```python
from build123d import *

# Parameters (mm, degrees)
BOSS_EXTRUDE1_DEPTH = 152.4
BOSS_EXTRUDE2_DEPTH = 173.99
CUT_EXTRUDE1_DEPTH  = 232.798485112
BOSS_EXTRUDE3_DEPTH = 2.54
CUT_EXTRUDE2_DEPTH  = 247.386546305
FILLET1_R           = 2.54


with BuildPart() as part:
    # Sketch1 → Boss-Extrude1 (new body)
    with BuildSketch(Plane.XY):
        Polygon((0, 0), (-173.99, 0), (-158.75, 15.24), (-152.4, 15.24), (-152.4, 2.54), (0, 2.54), align=None)
    extrude(amount=BOSS_EXTRUDE1_DEPTH)

    # Sketch2 → Boss-Extrude2 (add, through all)
    with BuildSketch(Plane(origin=(0, 0, 0), x_dir=(0, 0, -1), z_dir=(1, 0, 0))):
        Polygon((-152.4, 2.54), (-152.4, 15.24), (-158.75, 15.24), (-173.99, 0), (-152.4, 0), align=None)
    extrude(amount=-BOSS_EXTRUDE2_DEPTH)

    # Sketch3 → Cut-Extrude1 (cut, through all)
    with BuildSketch(Plane(origin=(0, 0, 152.4), x_dir=(-1, 0, 0), z_dir=(0, 0, -1))):
        Polygon((158.75, 15.24), (173.99, 0), (173.99, 15.24), align=None)
    extrude(amount=-CUT_EXTRUDE1_DEPTH, mode=Mode.SUBTRACT)

    # Sketch4 → Boss-Extrude3 (add, through all)
    with BuildSketch(Plane(origin=(0, 2.54, 0), x_dir=(1, 0, 0), z_dir=(0, 1, 0))):
        with BuildLine():
            ThreePointArc((-105.230385896, 0), (-114.3, 21.59), (-123.369614104, 0))
            Line((-123.369614104, 0), (-105.230385896, 0))
        make_face()
        with BuildLine():
            ThreePointArc((0, -47.169614104), (21.59, -38.1), (0, -29.030385896))
            Line((0, -29.030385896), (0, -47.169614104))
        make_face()
    extrude(amount=-BOSS_EXTRUDE3_DEPTH)

    # Sketch4<3> → Cut-Extrude2 (cut, through all)
    with BuildSketch(Plane(origin=(0, 2.54, 0), x_dir=(1, 0, 0), z_dir=(0, 1, 0))):
        with BuildLine():
            Line((-29.030385896, 0), (-47.169614104, 0))
            ThreePointArc((-47.169614104, 0), (-38.1, -21.59), (-29.030385896, 0))
        make_face()
        with BuildLine():
            Line((0, -123.369614104), (0, -105.230385896))
            ThreePointArc((0, -105.230385896), (-21.59, -114.3), (0, -123.369614104))
        make_face()
    extrude(amount=-CUT_EXTRUDE2_DEPTH, mode=Mode.SUBTRACT)

    # Fillet1
    fillet1_edges = [part.edges().sort_by_distance(p)[0] for p in [
        (-123.369614104, 1.27, 0),
        (-105.230385896, 1.27, 0),
        (0, 1.27, 29.030385896),
        (0, 1.27, 47.169614104),
        (-47.169614104, 1.27, 0),
        (-29.030385896, 1.27, 0),
        (0, 1.27, 105.230385896),
        (0, 1.27, 123.369614104),
    ]]
    fillet(fillet1_edges, radius=FILLET1_R)


solid = part.part
```
Geometry: final body of the model. Coordinates: model frame, mm. A direction names the side the tool comes from. Coordinates: 2 decimals unless noted, no trailing zeros. Order: outer loops, then holes, each group sorted by start corner. A loop starts at its lowest first (then second) coordinate and runs counter-clockwise, first axis right, second up.
Item 1: Access query for faces 1 (the face through (0, 6, 156)), 2 (the face through (-156, 6, 0)), 3 (the face through (21.585, 1.288, 38.456)), 4 (the face through (-152.4, 9, 75)). Directions: +Z, -Z, +X, -X, +Y, -Y. A direction counts if a zero-diameter tool reaches every point of the face in a straight line with its end or side. Return the directions, or none.
Answer:
face 1: +Z, +X, +Y, -Y
face 2: -Z, -X, +Y, -Y
face 3: +Y, -Y
face 4: -Z, +X, +Y
Item 2: Contact query for flat-ended pins moving along their axis: P1, Ø6, axis at x = -33.5, y = 8.5, coming from the +Z side; P2, Ø7.5, axis at x = -161, y = 11.5, coming from the -Z side; P3, Ø0.8, axis at y = 1, z = 77.5, coming from the +X side. Output: stop coordinate, or through.
Answer:
P1: stops at z = 168.49
P2: stops at z = 0
P3: stops at x = 0
Item 3: Section query D-D (z = 38.1). Output: boundary loops of the cut face in (x, y), then the cut area to 3 significant figures.
Answer:
outline: (-173.99, 0) - (21.59, 0) - (21.59, 2.54) - (-152.4, 2.54) - (-152.4, 15.24) - (-158.75, 15.24) - close
area: 655 mm2
Item 4: Material intervals for line 1 along Y through (x, z) = (-1, 39); line 2 along X through (y, z) = (1.35, 8.89); line 3 along Z through (x, y) = (-126, 2.5), sorted ascending.
Answer:
line 1: y = 0 to 2.54
line 2: x = -172.64 to -50.8, -25.4 to 0
line 3: z = -13.83 to -3.95, -1.19 to 171.49
Item 5: Section query A-A (z = 8.89). Output: boundary loops of the cut face in (x, y).
Answer:
outline: (-173.99, 0) - (-50.8, 0) - (-50.8, 2.54) - (-152.4, 2.54) - (-152.4, 15.24) - (-158.75, 15.24) - close; (-25.4, 0) - (0, 0) - (0, 2.54) - (-25.4, 2.54) - close
Item 6: Draft query along Z for faces 5 (the face through (-166.26, 7.73, 85.78)), 6 (the face through (-75, 9, 152.4)), 7 (the face through (-38.456, 1.288, 21.585)). Return one class per face: released by +Z, released by -Z, zero draft, split by the parting line, or undercut.
Answer:
face 5: zero draft
face 6: released by -Z
face 7: undercut
Item 7: Section query C-C (x = -134.5). Output: boundary loops of the cut face in (y, z).
Answer:
outline: (0, 0) - (2.54, 0) - (2.54, 152.4) - (15.24, 152.4) - (15.24, 158.75) - (0, 173.99) - close
Item 8: Section query B-B (x = -8.89). Output: boundary loops of the cut face in (y, z), then the cut area to 3 significant figures.
Answer:
outline: (0, 0) - (2.54, 0) - (2.54, 101.6) - (0, 101.6) - close; (0, 127) - (2.54, 127) - (2.54, 152.4) - (15.24, 152.4) - (15.24, 158.75) - (0, 173.99) - close
area: 535 mm2
